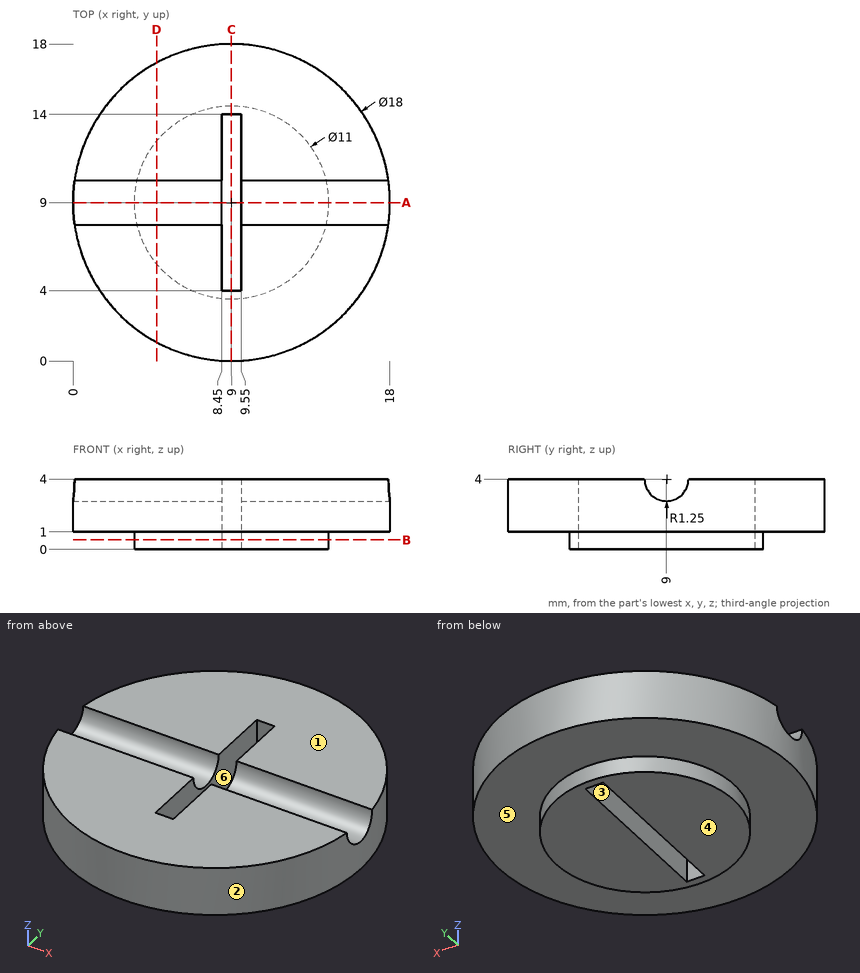
For this review, use the dimensioned drawing (mm, ordinates from the lowest corner) and the shaded views. A direction names the side the tool comes from. Round coordinates to 2 decimals unless told otherwise and drop trailing zeros. Write each loop counter-clockwise with the first axis right and the second up, starting at its lowest first coordinate (ties: lowest second). Pieces come first, ordered by that corner, then holes. Notation, with made-up numbers: (-16.75, -28) - (0.25, -28) arc R19 ccw to (0.25, -16) - close; hole circle Ø11 at (74.25, 45). An arc over 180 degrees is marked (long way). Answer as a JSON object with one key per item and string values.
1. To check wall thickness, follow line 1 along Y through (x, z) = (8.75, 1.3); line 2 along Z through (x, y) = (15.5, 3.75); line 3 along Y through (x, z) = (1, 3.2). State the ranges of each line that lie inside material, in increasing order.
Response values:
{"line 1": "y = 0 to 4, 14 to 18", "line 2": "z = 1 to 4", "line 3": "y = 4.88 to 8.04, 9.96 to 13.12"}
2. We need section C-C on x = 9. Give the boundary of the cut face in (y, z).
Response values:
{"outline": "(0, 1) - (3.5, 1) - (3.5, 0) - (4, 0) - (4, 4) - (0, 4) - close; (14, 0) - (14.5, 0) - (14.5, 1) - (18, 1) - (18, 4) - (14, 4) - close"}
3. We need section D-D on x = 4.75. Give the boundary of the cut face in (y, z), then the cut area to 3 significant figures.
Response values:
{"outline": "(1.07, 1) - (5.51, 1) - (5.51, 0) - (12.49, 0) - (12.49, 1) - (16.93, 1) - (16.93, 4) - (10.25, 4) arc R1.25 cw to (7.75, 4) - (1.07, 4) - close", "area": "52.1 mm2"}
4. We need section A-A on y = 9. Give the boundary of the cut face in (x, z).
Response values:
{"outline": "(0, 1) - (3.5, 1) - (3.5, 0) - (8.45, 0) - (8.45, 2.75) - (0, 2.75) - close; (9.55, 0) - (14.5, 0) - (14.5, 1) - (18, 1) - (18, 2.75) - (9.55, 2.75) - close"}
5. Tool access review of the marked faces 4, 5 and 6: name each direction out of +Z, -Z, +X, -X, +Y, -Y from which nothing blocks a thin tool from reaching the whole face with its end or side.
Response values:
{"face 4": "-Z, +X, -X, +Y, -Y", "face 5": "-Z", "face 6": "+Z, -Z"}
6. We need section B-B on z = 0.55. Give the boundary of the cut face in (x, y).
Response values:
{"outline": "circle Ø11 at (9, 9); hole (8.45, 4) - (9.55, 4) - (9.55, 14) - (8.45, 14) - close"}
7. Draft analysis for pull direction X (two halves, no side actions). For the marked faces 1, 2 and 3, state which applies: +X half, -X half, draft (parallel to the pull), parting line (faces both ways), or undercut.
Response values:
{"face 1": "draft", "face 2": "parting line", "face 3": "undercut"}
8. For pin 1 Ø2 at (y, z) = (10.5, 1.5) entering from -X; pin 2 Ø2 at (x, y) = (10.5, 2.5) entering from -Z; pin 3 Ø2 at (y, z) = (9.5, 1.5) entering from +X; pin 4 Ø1.2 at (y, z) = (7, 2.5) entering from -X, all flat-tipped, find the tip position at first contact; note any pin that passes through.
Response values:
{"pin 1": "stops at x = 0.01", "pin 2": "stops at z = 1", "pin 3": "stops at x = 18", "pin 4": "stops at x = 0.11"}
